Part model, mm, in its own coordinate system. Face numbers are marked on the shaded views. A direction names the side the tool comes from. Coordinates: 2 decimals unless noted, no trailing zeros. Write each loop counter-clockwise with the first axis right and the second up, starting at its lowest first coordinate (ties: lowest second). Pieces come first, ordered by that corner, then holes. Notation, with made-up numbers: (51.25, 83) - (91.25, 83) arc R7 cw to (91.25, 94) - close; hole circle Ø3 at (27, -11.75). An arc over 180 degrees is marked (long way). Use a Markdown table: item, result.
```python
from build123d import *

# Parameters (mm, degrees)
SKETCH_1_R      = 4.25
EXTRUDE_1_DEPTH = 5
SKETCH_2_R      = 2.5
EXTRUDE_2_DEPTH = 15
FILLET_1_R      = 1


with BuildPart() as part:
    # ｽｹｯﾁ1 → ﾎﾞｽ - 押し出し1 (new body)
    with BuildSketch(Plane.XY):
        Circle(SKETCH_1_R)
    extrude(amount=EXTRUDE_1_DEPTH)

    # ｽｹｯﾁ2 → ﾎﾞｽ - 押し出し2 (add)
    with BuildSketch(Plane.XY.offset(5)):
        Circle(SKETCH_2_R)
    extrude(amount=EXTRUDE_2_DEPTH)

    # ﾌｨﾚｯﾄ1
    fillet_1_edges = [part.edges().sort_by_distance(p)[0] for p in [
        (-4.25, 0, 0),
    ]]
    fillet(fillet_1_edges, radius=FILLET_1_R)


solid = part.part
```
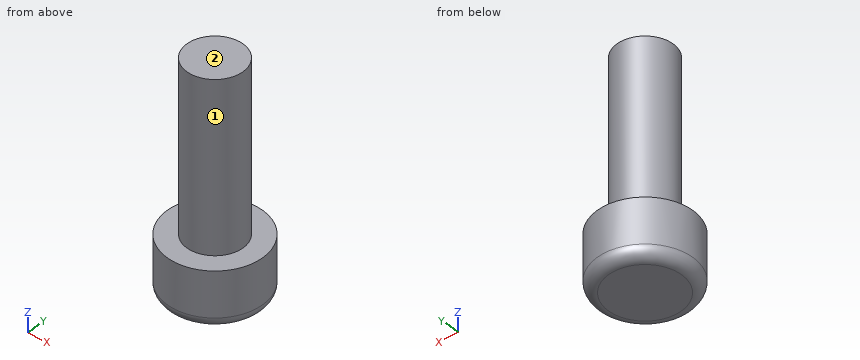
Item 1: Band-saw the part on C-C, the plane z = 15. Give the cut face in (x, y).
From the geometry:
| item | result |
|---|---|
| outline | circle Ø5 at (0, 0) |
Item 2: Drop a flat-ended pin along its axis: P1, Ø2, axis at y = -1, z = 15, coming from the +X side. Give the stop position or say it passes through.
From the geometry:
| item | result |
|---|---|
| P1 | x = 2.5 |
Item 3: Drill centre lines: probe 1 along Z at (x, y) = (-3, 1.25); probe 2 along X at (y, z) = (-0.25, 12.25); probe 3 along X at (y, z) = (-0.5, 15). Where is each one in solid material? Low to high.
From the geometry:
| item | result |
|---|---|
| probe 1 | 0 to 5 |
| probe 2 | -2.49 to 2.49 |
| probe 3 | -2.45 to 2.45 |
Item 4: Band-saw the part on A-A, the plane y = 0. Give the cut face in (x, z), then the cut area to 3 significant figures.
From the geometry:
| item | result |
|---|---|
| outline | (-4.25, 1) arc R1 ccw to (-3.25, 0) - (3.25, 0) arc R1 ccw to (4.25, 1) - (4.25, 5) - (2.5, 5) - (2.5, 20) - (-2.5, 20) - (-2.5, 5) - (-4.25, 5) - close |
| area | 117 mm^2 |
Item 5: Band-saw the part on D-D, the plane z = 4.5. Give the cut face in (x, y), then the cut area to 3 significant figures.
From the geometry:
| item | result |
|---|---|
| outline | circle Ø8.5 at (0, 0) |
| area | 56.7 mm^2 |
Item 6: Which spindle directions (+Z, -Z, +X, -X, +Y, -Y) get a long thin tool onto all of the face, cutting with end or side? Do the marked faces 1 and 2. Say none if no direction does.
From the geometry:
| item | result |
|---|---|
| face 1 | +Z |
| face 2 | +Z, +X, -X, +Y, -Y |
